from build123d import *

# Parameters (mm, degrees)
SKETCH1_R           = 7
BOSS_EXTRUDE1_DEPTH = 3
SKETCH1_3_R         = 4
BOSS_EXTRUDE2_DEPTH = 30
CHAMFER1_SIZE       = 1
CUT_EXTRUDE1_REACH  = 34.711
SKETCH2_R           = 0.95


with BuildPart() as part:
    # Sketch1 → Boss-Extrude1 (new body)
    with BuildSketch(Plane(origin=(0, 0, 0), x_dir=(1, 0, 0), z_dir=(0, 1, 0))):
        with Locations(Location((0, 0, 0), (0, 0, 270))):
            Circle(SKETCH1_R)
    extrude(amount=-BOSS_EXTRUDE1_DEPTH)

    # Sketch1_3 → Boss-Extrude2 (add)
    with BuildSketch(Plane(origin=(0, 0, 0), x_dir=(1, 0, 0), z_dir=(0, 1, 0))):
        with Locations(Location((0, 0, 0), (0, 0, 270))):
            Circle(SKETCH1_3_R)
    extrude(amount=BOSS_EXTRUDE2_DEPTH)

    # Chamfer1
    chamfer1_edges = [part.edges().sort_by_distance(p)[0] for p in [
        (0, -3, -7),
    ]]
    chamfer(chamfer1_edges, length=CHAMFER1_SIZE)

    # Sketch2 → Cut-Extrude1 (cut, up to next)
    with BuildSketch(Plane.ZY.offset(4), mode=Mode.PRIVATE) as cut_extrude1_sk1:
        with Locations((0, 28)):
            Circle(SKETCH2_R)
    cut_extrude1_tool1 = extrude(cut_extrude1_sk1.sketch, amount=-CUT_EXTRUDE1_REACH, mode=Mode.PRIVATE) & part.part
    add(cut_extrude1_tool1.solids().sort_by_distance((-4, 28, 0))[0], mode=Mode.SUBTRACT)


solid = part.part
Part model, mm, in its own coordinate system. Round coordinates to 2 decimals unless told otherwise and drop trailing zeros. Loops run counter-clockwise (first coordinate to the right, second up) from the corner with the lowest first, then second, coordinate; pieces in that order, holes last. Notation, with made-up numbers: (15, -16.5) - (55, -16.5) arc R18 cw to (55, -3.5) - close; hole circle Ø7 at (-26, 19). An arc over 180 degrees is marked (long way). Answer as a JSON object with one key per item and string values.
Item 1: Band-saw the part on B-B on x = 0. List the corners of the cut face in (y, z), plus the area to 3 significant figures.
Output:
{"outline": "(-3, -6) - (-2, -7) - (0, -7) - (0, -4) - (30, -4) - (30, 4) - (0, 4) - (0, 7) - (-2, 7) - (-3, 6) - close; hole circle Ø1.9 at (28, 0)", "area": "278 mm2"}
Item 2: Band-saw the part on C-C on y = 24. List the corners of the cut face in (x, z).
Output:
{"outline": "circle Ø8 at (0, 0)"}
Item 3: Pin check, flat tips, straight feed: pin 1 (5 mm diameter, centred on y = 22, z = -3, fed in from -X); pin 2 (3 mm diameter, centred on y = 24.5, z = 2, fed in from +X); pin 3 (6 mm diameter, centred on x = 3.5, y = 8.5, fed in from +Z). Stop position of each tip, or through.
Output:
{"pin 1": "x = -3.97", "pin 2": "x = 3.97", "pin 3": "z = 3.97"}
Item 4: Wall check: L1, parallel to Y at x = -0.75, z = 0; L2, parallel to Z at x = -0.25, y = 28; L3, parallel to Y at x = -0.75, z = -4.25. Give the ranges that are in metal, low to high.
Output:
{"L1": "-3 to 27.05, 28.95 to 30", "L2": "-3.99 to -0.95, 0.95 to 3.99", "L3": "-3 to 0"}
Item 5: Pull direction Z, two halves, no side cores. Call faces 1 (the face through (-0.054, 27.073, -0.206)), 2 (the face through (-3, 0, 3)), 3 (the face through (-1.532, 14.79, 3.695)): pulls with the +Z half, pulls with the -Z half, needs draft (parallel to the pull), parting line crosses it, or undercut.
Output:
{"face 1": "undercut", "face 2": "needs draft", "face 3": "parting line crosses it"}
Item 6: Band-saw the part on A-A on z = 0. List the corners of the cut face in (x, y).
Output:
{"outline": "(-7, -2) - (-6, -3) - (6, -3) - (7, -2) - (7, 0) - (4, 0) - (4, 27.05) - (-4, 27.05) - (-4, 0) - (-7, 0) - close; (-4, 28.95) - (4, 28.95) - (4, 30) - (-4, 30) - close"}
Item 7: Band-saw the part on D-D on y = 28. List the corners of the cut face in (x, z), plus the area to 3 significant figures.
Output:
{"outline": "(-3.89, -0.95) arc R4 ccw to (3.89, -0.95) - close; (-3.89, 0.95) - (3.89, 0.95) arc R4 ccw to start", "area": "35.2 mm2"}
